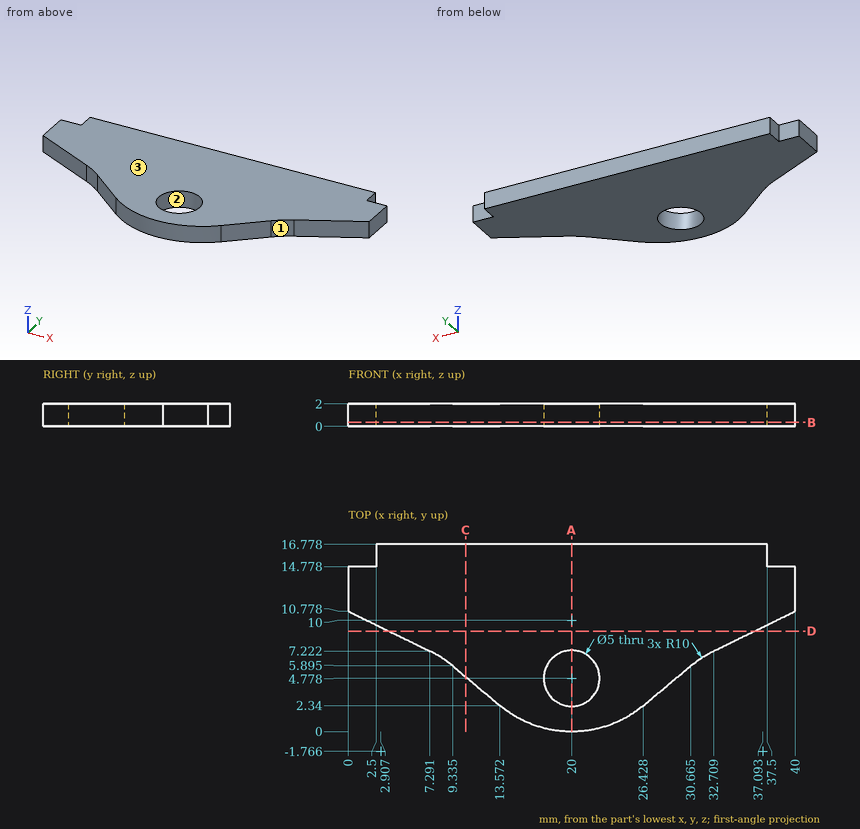
Here's the drawing with two shaded views (mm, measured from the low corner). I have some questions. Round coordinates to 2 decimals unless told otherwise and drop trailing zeros. Loops run counter-clockwise (first coordinate to the right, second up) from the corner with the lowest first, then second, coordinate; pieces in that order, holes last. Notation, with made-up numbers: M 0,40 L 58,40 A15 cw 58,62 Z; hole C 52,50.5 d9. An arc over 180 degrees is marked long. Put each result on its own line as item: value.
Q1. Imagine slicing it at A-A (x = 20). Write out the boundary of the cut face in (y, z).
Check result:
outline: M 0,0 L 2.28,0 L 2.28,2 L 0,2 Z; M 7.28,0 L 16.78,0 L 16.78,2 L 7.28,2 Z
Q2. I need wall thicknesses on probe 1 along Y at (x, z) = (20, 0.95); probe 2 along X at (y, z) = (3, 1.25) (1 decimal); probe 3 along X at (y, z) = (15.75, 1.9). Which ranges of each line are inside material? Lowest first, please.
Check result:
probe 1: 0 to 2.28, 7.28 to 16.78
probe 2: 12.8 to 18.2, 21.8 to 27.2
probe 3: 2.5 to 37.5
Q3. Imagine slicing it at C-C (x = 10.5). Write out the boundary of the cut face in (y, z).
Check result:
outline: M 4.92,0 L 16.78,0 L 16.78,2 L 4.92,2 Z
Q4. Imagine slicing it at D-D (y = 9). Write out the boundary of the cut face in (x, z).
Check result:
outline: M 3.65,0 L 36.35,0 L 36.35,2 L 3.65,2 Z
Q5. Imagine slicing it at B-B (z = 0.35). Write out the boundary of the cut face in (x, y) (1 decimal).
Check result:
outline: M 0,10.8 L 7.3,7.2 A10 cw 9.3,5.9 L 13.6,2.3 A10 ccw 26.4,2.3 L 30.7,5.9 A10 cw 32.7,7.2 L 40,10.8 L 40,14.8 L 37.5,14.8 L 37.5,16.8 L 2.5,16.8 L 2.5,14.8 L 0,14.8 Z; hole C 20,4.8 d5
Q6. Thinking about a two-plate mould opening in Y: for the marked faces 1, 2 and 3, which applies, released by +Y, released by -Y, zero draft, split by the parting line, or undercut?
Check result:
face 1: released by -Y
face 2: undercut
face 3: zero draft
Q7. For pin 1 (0.6 mm diameter, centred on y = 16.5, z = 1, fed in from -X); pin 2 (0.6 mm diameter, centred on x = 1.5, z = 1, fed in from +Y), each with a flat end and sliding along its axis, tell me the tip position at first contact or that it passes through.
Check result:
pin 1: x = 2.5
pin 2: y = 14.78
